Read the model definition and answer for the solid it produces. Units are mm, in the model's axes. A direction names the side the tool comes from. Give positions to 0.01 mm unless a question says otherwise; leave off trailing zeros. Order: outer loops, then holes, each group sorted by start corner. A loop starts at its lowest first (then second) coordinate and runs counter-clockwise, first axis right, second up. Notation, with made-up numbers: M 27,84 L 86,84 A14 cw 86,90 Z; hole C 17,81 d9. An arc over 180 degrees is marked long. One line per item, written item: value.
from build123d import *
from build123d.topology import SkipClean

# Parameters (mm, degrees)
ESBO_O1_R                = 11.15
RESSALTO_EXTRUS_O1_DEPTH = 15
ESBO_O2_R                = 22.5
RESSALTO_EXTRUS_O2_DEPTH = 4
RESSALTO_EXTRUS_O6_START = -8
ESBO_O5_R                = 11.15
ESBO_O5_R_2              = 8
RESSALTO_EXTRUS_O6_DEPTH = 8
RESSALTO_EXTRUS_O7_START = 4
ESBO_O7_R                = 14.2
ESBO_O7_R_2              = 11.15
RESSALTO_EXTRUS_O7_DEPTH = 4
RESSALTO_EXTRUS_O8_START = 4
ESBO_O8_R                = 11.15
ESBO_O8_R_2              = 8
RESSALTO_EXTRUS_O8_DEPTH = 4
RESSALTO_EXTRUS_O9_DEPTH = 7
CORTE_EXTRUS_O2_START    = -15
CORTE_EXTRUS_O2_DEPTH    = 15
CORTE_EXTRUS_O3_START    = -11
CORTE_EXTRUS_O3_DEPTH    = 11


with BuildPart() as part:
    # Esbo_o1 → Ressalto-extrus_o1 (new body)
    with BuildSketch(Plane.XY):
        with BuildLine():
            Line((-2.5, 18), (-2.5, 13.978197309))
            ThreePointArc((-2.5, 13.978197309), (-10.040916293, 10.040916293), (-13.978197309, 2.5))
            Line((-13.978197309, 2.5), (-18, 2.5))
            Line((-18, 2.5), (-18, -2.5))
            Line((-18, -2.5), (-13.978197309, -2.5))
            ThreePointArc((-13.978197309, -2.5), (-10.040916293, -10.040916293), (-2.5, -13.978197309))
            Line((-2.5, -13.978197309), (-2.5, -18))
            Line((-2.5, -18), (2.5, -18))
            Line((2.5, -18), (2.5, -13.978197309))
            ThreePointArc((2.5, -13.978197309), (10.040916293, -10.040916293), (13.978197309, -2.5))
            Line((13.978197309, -2.5), (18, -2.5))
            Line((18, -2.5), (18, 2.5))
            Line((18, 2.5), (13.978197309, 2.5))
            ThreePointArc((13.978197309, 2.5), (10.040916293, 10.040916293), (2.5, 13.978197309))
            Line((2.5, 13.978197309), (2.5, 18))
            Line((2.5, 18), (-2.5, 18))
        make_face()
        Circle(ESBO_O1_R, mode=Mode.SUBTRACT)
    extrude(amount=RESSALTO_EXTRUS_O1_DEPTH)

    # Esbo_o5 → Ressalto-extrus_o6 (add)
    with BuildSketch(Plane.XY.offset(15).offset(RESSALTO_EXTRUS_O6_START)):
        Circle(ESBO_O5_R)
        Circle(ESBO_O5_R_2, mode=Mode.SUBTRACT)
    extrude(amount=RESSALTO_EXTRUS_O6_DEPTH)



with BuildPart() as body_2:
    # Esbo_o2 → Ressalto-extrus_o2 (new body)
    # profile 1 of 5: a face of its own
    with SkipClean():  # the faces are left unmerged after this step: merging them gives an invalid solid
        with BuildSketch(Plane(origin=(0, 0, 0), x_dir=(-1, 0, 0), z_dir=(0, 0, -1))):
            Circle(ESBO_O2_R)
            with BuildLine():
                Line((2.5, 13.978197309), (2.5, 18))
                Line((2.5, 18), (-2.5, 18))
                Line((-2.5, 18), (-2.5, 13.978197309))
                ThreePointArc((-2.5, 13.978197309), (-10.040916293, 10.040916293), (-13.978197309, 2.5))
                Line((-13.978197309, 2.5), (-18, 2.5))
                Line((-18, 2.5), (-18, -2.5))
                Line((-18, -2.5), (-13.978197309, -2.5))
                ThreePointArc((-13.978197309, -2.5), (-10.040916293, -10.040916293), (-2.5, -13.978197309))
                Line((-2.5, -13.978197309), (-2.5, -18))
                Line((-2.5, -18), (2.5, -18))
                Line((2.5, -18), (2.5, -13.978197309))
                ThreePointArc((2.5, -13.978197309), (10.040916293, -10.040916293), (13.978197309, -2.5))
                Line((13.978197309, -2.5), (18, -2.5))
                Line((18, -2.5), (18, 2.5))
                Line((18, 2.5), (13.978197309, 2.5))
                ThreePointArc((13.978197309, 2.5), (10.040916293, 10.040916293), (2.5, 13.978197309))
            make_face(mode=Mode.SUBTRACT)
        # profile 2 of 5: a face of its own
        with BuildSketch(Plane(origin=(0, 0, 0), x_dir=(-1, 0, 0), z_dir=(0, 0, -1))):
            with BuildLine():
                Line((2.5, -18), (2.5, -13.978197309))
                ThreePointArc((2.5, -13.978197309), (0, -14.2), (-2.5, -13.978197309))
                Line((-2.5, -13.978197309), (-2.5, -18))
                Line((-2.5, -18), (2.5, -18))
            make_face()
        # profile 3 of 5: a face of its own
        with BuildSketch(Plane(origin=(0, 0, 0), x_dir=(-1, 0, 0), z_dir=(0, 0, -1))):
            with BuildLine():
                ThreePointArc((-13.978197309, -2.5), (-14.2, 0), (-13.978197309, 2.5))
                Line((-13.978197309, 2.5), (-18, 2.5))
                Line((-18, 2.5), (-18, -2.5))
                Line((-18, -2.5), (-13.978197309, -2.5))
            make_face()
        # profile 4 of 5: a face of its own
        with BuildSketch(Plane(origin=(0, 0, 0), x_dir=(-1, 0, 0), z_dir=(0, 0, -1))):
            with BuildLine():
                ThreePointArc((-2.5, 13.978197309), (0, 14.2), (2.5, 13.978197309))
                Line((2.5, 13.978197309), (2.5, 18))
                Line((2.5, 18), (-2.5, 18))
                Line((-2.5, 18), (-2.5, 13.978197309))
            make_face()
        # profile 5 of 5: a face of its own
        with BuildSketch(Plane(origin=(0, 0, 0), x_dir=(-1, 0, 0), z_dir=(0, 0, -1))):
            with BuildLine():
                Line((18, 2.5), (13.978197309, 2.5))
                ThreePointArc((13.978197309, 2.5), (14.2, 0), (13.978197309, -2.5))
                Line((13.978197309, -2.5), (18, -2.5))
                Line((18, -2.5), (18, 2.5))
            make_face()
        extrude(amount=RESSALTO_EXTRUS_O2_DEPTH)


with BuildPart() as part_1:
    with SkipClean():  # the faces are left unmerged after this step: merging them gives an invalid solid
        add(part.part)

        add(body_2.part)  # Ressalto-extrus_o7 merges body 2
        # Esbo_o7 → Ressalto-extrus_o7 (add)
        with BuildSketch(Plane(origin=(0, 0, 0), x_dir=(-1, 0, 0), z_dir=(0, 0, -1)).offset(RESSALTO_EXTRUS_O7_START)):
            Circle(ESBO_O7_R)
            with Locations(Location((0, 0, 0), (0, 0, 180))):
                Circle(ESBO_O7_R_2, mode=Mode.SUBTRACT)
        extrude(amount=-RESSALTO_EXTRUS_O7_DEPTH)

    # Esbo_o8 → Ressalto-extrus_o8 (add)
    with BuildSketch(Plane(origin=(0, 0, 7), x_dir=(-1, 0, 0), z_dir=(0, 0, -1)).offset(RESSALTO_EXTRUS_O8_START)):
        Circle(ESBO_O8_R)
        with Locations(Location((0, 0, 0), (0, 0, 180))):
            Circle(ESBO_O8_R_2, mode=Mode.SUBTRACT)
    extrude(amount=-RESSALTO_EXTRUS_O8_DEPTH)

    # Esbo_o9 → Ressalto-extrus_o9 (add)
    with BuildSketch(Plane.XY.offset(15)):
        with BuildLine():
            Line((-11.419478117, 5.324990098), (-8.609923977, 4.014873487))
            ThreePointArc((-8.609923977, 4.014873487), (0, 9.5), (8.609923977, 4.014873487))
            Line((8.609923977, 4.014873487), (11.419478117, 5.324990098))
            ThreePointArc((11.419478117, 5.324990098), (0, 12.6), (-11.419478117, 5.324990098))
        make_face()
        with BuildLine():
            Line((-11.419478117, -5.324990098), (-8.609923977, -4.014873487))
            ThreePointArc((-8.609923977, -4.014873487), (0, -9.5), (8.609923977, -4.014873487))
            Line((8.609923977, -4.014873487), (11.419478117, -5.324990098))
            ThreePointArc((11.419478117, -5.324990098), (0, -12.6), (-11.419478117, -5.324990098))
        make_face()
    extrude(amount=RESSALTO_EXTRUS_O9_DEPTH)

    # Esbo_o10 → Corte-extrus_o2 (cut)
    with BuildSketch(Plane.XY.offset(15).offset(CORTE_EXTRUS_O2_START)):
        with BuildLine():
            Line((-2.5, 18), (-2.5, 13.978197309))
            ThreePointArc((-2.5, 13.978197309), (-10.040916293, 10.040916293), (-13.978197309, 2.5))
            Line((-13.978197309, 2.5), (-18, 2.5))
            Line((-18, 2.5), (-18, -2.5))
            Line((-18, -2.5), (-13.978197309, -2.5))
            ThreePointArc((-13.978197309, -2.5), (-10.040916293, -10.040916293), (-2.5, -13.978197309))
            Line((-2.5, -13.978197309), (-2.5, -18))
            Line((-2.5, -18), (2.5, -18))
            Line((2.5, -18), (2.5, -13.978197309))
            ThreePointArc((2.5, -13.978197309), (10.040916293, -10.040916293), (13.978197309, -2.5))
            Line((13.978197309, -2.5), (18, -2.5))
            Line((18, -2.5), (18, 2.5))
            Line((18, 2.5), (13.978197309, 2.5))
            ThreePointArc((13.978197309, 2.5), (10.040916293, 10.040916293), (2.5, 13.978197309))
            Line((2.5, 13.978197309), (2.5, 18))
            Line((2.5, 18), (-2.5, 18))
        make_face()
        with BuildLine():
            Line((11.419478117, -5.324990098), (8.609923977, -4.014873487))
            ThreePointArc((8.609923977, -4.014873487), (0, -9.5), (-8.609923977, -4.014873487))
            Line((-8.609923977, -4.014873487), (-11.419478117, -5.324990098))
            ThreePointArc((-11.419478117, -5.324990098), (0, -12.6), (11.419478117, -5.324990098))
        make_face(mode=Mode.SUBTRACT)
        with BuildLine():
            Line((8.609923977, 4.014873487), (11.419478117, 5.324990098))
            ThreePointArc((11.419478117, 5.324990098), (0, 12.6), (-11.419478117, 5.324990098))
            Line((-11.419478117, 5.324990098), (-8.609923977, 4.014873487))
            ThreePointArc((-8.609923977, 4.014873487), (0, 9.5), (8.609923977, 4.014873487))
        make_face(mode=Mode.SUBTRACT)
    extrude(amount=CORTE_EXTRUS_O2_DEPTH, mode=Mode.SUBTRACT)

    # Esbo_o11 → Corte-extrus_o3 (cut)
    with BuildSketch(Plane.XY.offset(22).offset(CORTE_EXTRUS_O3_START)):
        with BuildLine():
            Line((11.419478117, -5.324990098), (8.609923977, -4.014873487))
            ThreePointArc((8.609923977, -4.014873487), (0, -9.5), (-8.609923977, -4.014873487))
            Line((-8.609923977, -4.014873487), (-11.419478117, -5.324990098))
            ThreePointArc((-11.419478117, -5.324990098), (0, -12.6), (11.419478117, -5.324990098))
        make_face()
        with BuildLine():
            Line((8.609923977, 4.014873487), (11.419478117, 5.324990098))
            ThreePointArc((11.419478117, 5.324990098), (0, 12.6), (-11.419478117, 5.324990098))
            Line((-11.419478117, 5.324990098), (-8.609923977, 4.014873487))
            ThreePointArc((-8.609923977, 4.014873487), (0, 9.5), (8.609923977, 4.014873487))
        make_face()
    extrude(amount=CORTE_EXTRUS_O3_DEPTH, mode=Mode.SUBTRACT)


solid = part_1.part
1) Each of these flat-tipped pins is pushed along its axis until it touches: pin 1 Ø13.5 at (x, y) = (0, 0) entering from -Z; pin 2 Ø5 at (x, y) = (15, -3) entering from +Z; pin 3 Ø8 at (x, z) = (13.5, 1) entering from -Y; pin 4 Ø2 at (y, z) = (-12.5, 4.5) entering from +X. Where does it stop, or does it pass through?
Reported:
pin 1: passes through
pin 2: stops at z = 0
pin 3: stops at y = -20.34
pin 4: stops at x = 5.15
2) Find section B-B, the plane x = 0. Write down the section's boundary in (y, z), plus the area to 3 significant figures.
Reported:
outline: M -22.5,-4 L -11.15,-4 L -11.15,3 L -9.5,3 L -9.5,11 L -12.6,11 L -12.6,0 L -22.5,0 Z; M 9.5,3 L 11.15,3 L 11.15,-4 L 22.5,-4 L 22.5,0 L 12.6,0 L 12.6,11 L 9.5,11 Z
area: 149 mm^2
3) Find section A-A, the plane y = 0. Write down the section's boundary in (x, z).
Reported:
outline: M -22.5,-4 L -11.15,-4 L -11.15,0 L -22.5,0 Z; M 11.15,-4 L 22.5,-4 L 22.5,0 L 11.15,0 Z
4) Find section C-C, the plane z = 8. Write down the section's boundary in (x, y) (3 decimals).
Reported:
outline: M -11.419,-5.325 A12.6 ccw 11.419,-5.325 L 8.61,-4.015 A9.5 cw -8.61,-4.015 Z; M -11.419,5.325 L -8.61,4.015 A9.5 cw 8.61,4.015 L 11.419,5.325 A12.6 ccw Z
5) Find section D-D, the plane y = -7.5. Write down the section's boundary in (x, z), plus the area to 3 significant figures.
Reported:
outline: M -21.21,-4 L -8.25,-4 L -8.25,3 L -5.83,3 L -5.83,11 L -10.12,11 L -10.12,0 L -21.21,0 Z; M 5.83,3 L 8.25,3 L 8.25,-4 L 21.21,-4 L 21.21,0 L 10.12,0 L 10.12,11 L 5.83,11 Z
area: 184 mm^2
6) Consider probe 1 along Y at (x, z) = (0, -1); probe 2 along Z at (x, y) = (-6, -19); probe 3 along Y at (x, z) = (-8, -0.5). Determine where each line is inside the solid, lowest interval first.
Reported:
probe 1: y = -22.5 to -11.15, 11.15 to 22.5
probe 2: z = -4 to 0
probe 3: y = -21.03 to -7.77, 7.77 to 21.03
7) Which of the six approach directions +Z, -Z, +X, -X, +Y, -Y give full straight-line access (tool end or side, diameter ignored) to faces 1 (the face through (-9.995, -4.661, 6.645)), 2 (the face through (0.2, 12.6, 5.4)), 3 (the face through (0, -10, 3)), 4 (the face through (10.034, -4.679, 6.645))?
Reported:
face 1: +Z, -X
face 2: +Z, +Y
face 3: -Z
face 4: +Z, +X
